Here's how the part is built. I have some questions about the finished solid (model axes, mm). A direction names the side the tool comes from. Round coordinates to 2 decimals unless told otherwise and drop trailing zeros. Write each loop counter-clockwise with the first axis right and the second up, starting at its lowest first coordinate (ties: lowest second). Pieces come first, ordered by that corner, then holes. Notation, with made-up numbers: (6, 79) -> (12, 79) arc R22 cw to (12, 117) -> close; hole circle Ø9 at (41.5, -30.75). An arc over 180 degrees is marked (long way). Answer in a Markdown table with one row per item.
from build123d import *

# Parameters (mm, degrees)
BOSS_EXTRUDE1_DEPTH = 12.5
SKETCH2_R           = 2
SKETCH2_R_2         = 0.5
BOSS_EXTRUDE2_DEPTH = 0.5
SKETCH2_2_R         = 0.5
BOSS_EXTRUDE3_DEPTH = 3
SKETCH2_4_R         = 2
BOSS_EXTRUDE4_DEPTH = 13.5
CUT_EXTRUDE1_START  = 12.5
SKETCH4_W           = 1.5
SKETCH4_H           = 2
CUT_EXTRUDE1_DEPTH  = 2
BOSS_EXTRUDE5_START = 12.5
SKETCH5_W           = 0.2
SKETCH5_H           = 1.5
BOSS_EXTRUDE5_DEPTH = 1.5
FILLET1_R           = 0.5
CUT_EXTRUDE2_START  = 12.5
CUT_EXTRUDE2_DEPTH  = 1


with BuildPart() as part:
    # Sketch1 → Boss-Extrude1 (new body)
    with BuildSketch(Plane.XY):
        with BuildLine():
            Line((-3, -4), (3, -4))
            ThreePointArc((3, -4), (5, 0), (3, 4))
            Line((3, 4), (-3, 4))
            ThreePointArc((-3, 4), (-5, 0), (-3, -4))
        make_face()
    extrude(amount=BOSS_EXTRUDE1_DEPTH)

    # Sketch2 → Boss-Extrude2 (add)
    with BuildSketch(Plane.XY):
        Circle(SKETCH2_R)
        Circle(SKETCH2_R_2, mode=Mode.SUBTRACT)
    extrude(amount=-BOSS_EXTRUDE2_DEPTH)

    # Sketch2<2> → Boss-Extrude3 (add)
    with BuildSketch(Plane.XY):
        Circle(SKETCH2_2_R)
    extrude(amount=-BOSS_EXTRUDE3_DEPTH)

    # Sketch2<4> → Boss-Extrude4 (add)
    with BuildSketch(Plane.XY):
        Circle(SKETCH2_4_R)
    extrude(amount=BOSS_EXTRUDE4_DEPTH)

    # Sketch4 → Cut-Extrude1 (cut)
    with BuildSketch(Plane.XY.offset(CUT_EXTRUDE1_START)):
        with Locations((0, 4)):
            Rectangle(SKETCH4_W, SKETCH4_H)
        with Locations((0, -4)):
            Rectangle(SKETCH4_W, SKETCH4_H)
    extrude(amount=-CUT_EXTRUDE1_DEPTH, mode=Mode.SUBTRACT)

    # Sketch5 → Boss-Extrude5 (add)
    with BuildSketch(Plane.XY.offset(BOSS_EXTRUDE5_START)):
        with Locations((3.1, 0)):
            Rectangle(SKETCH5_W, SKETCH5_H)
        with Locations((-3.1, 0)):
            Rectangle(SKETCH5_W, SKETCH5_H)
    extrude(amount=BOSS_EXTRUDE5_DEPTH)

    # Fillet1
    fillet1_edges = [part.edges().sort_by_distance(p)[0] for p in [
        (3.1, -0.75, 14),
        (3.1, 0.75, 14),
        (-3.1, -0.75, 14),
        (-3.1, 0.75, 14),
    ]]
    fillet(fillet1_edges, radius=FILLET1_R)

    # Sketch6 → Cut-Extrude2 (cut)
    with BuildSketch(Plane.XY.offset(CUT_EXTRUDE2_START)):
        with BuildLine():
            Line((-3, -4), (3, -4))
            ThreePointArc((3, -4), (5, 0), (3, 4))
            Line((3, 4), (-3, 4))
            ThreePointArc((-3, 4), (-5, 0), (-3, -4))
        make_face()
        with BuildLine():
            Line((-2.993325909, -3.98), (2.993325909, -3.98))
            ThreePointArc((2.993325909, -3.98), (4.98, 0), (2.993325909, 3.98))
            Line((2.993325909, 3.98), (-2.993325909, 3.98))
            ThreePointArc((-2.993325909, 3.98), (-4.98, 0), (-2.993325909, -3.98))
        make_face(mode=Mode.SUBTRACT)
    extrude(amount=-CUT_EXTRUDE2_DEPTH, mode=Mode.SUBTRACT)


solid = part.part
1) I need wall thicknesses on line 1 (Z direction, x = -1, y = 2.25); line 2 (Y direction, x = 0, z = -1.5); line 3 (Y direction, x = 4, z = 10). Which ranges of each line are inside material? Lowest first, please. Write a range as [from, to].
Response:
| item | result |
|---|---|
| line 1 | z = [0, 12.5] |
| line 2 | y = [-0.5, 0.5] |
| line 3 | y = [-3, 3] |
2) For pin 1 (1.5 mm diameter, centred on y = -3, z = 3, fed in from -X); pin 2 (0.8 mm diameter, centred on y = 0, z = 13, fed in from +X); pin 3 (0.5 mm diameter, centred on x = 1.5, z = 12, fed in from -Y); pin 4 (5 mm diameter, centred on x = -3.5, z = 11.5, fed in from +Y), each with a flat end and sliding along its axis, tell me the tip position at first contact or that it passes through.
Response:
| item | result |
|---|---|
| pin 1 | stops at x = -4.47 |
| pin 2 | stops at x = 3.2 |
| pin 3 | stops at y = -3.98 |
| pin 4 | stops at y = 4 |
3) We'd pull the mould along X, two halves only. Please class faces 1 (the face through (-3.2, 0, 13)), 2 (the face through (4.98, -0.06, 12.01)), 3 (the face through (0, -3.5, 10.5)), 4 (the face through (-0.108, -0.488, -1.732)): +X half, -X half, draft (parallel to the pull), parting line (faces both ways), or undercut.
Response:
| item | result |
|---|---|
| face 1 | -X half |
| face 2 | +X half |
| face 3 | undercut |
| face 4 | parting line |
4) I want a section at C-C, the plane z = 5. List the corners of the cut face in (x, y) for me, and give its area (3 significant figures).
Response:
| item | result |
|---|---|
| outline | (-3, -4) -> (3, -4) arc R5 ccw to (3, 4) -> (-3, 4) arc R5 ccw to start |
| area | 70.4 mm^2 |
5) I want a section at A-A, the plane x = 0. List the corners of the cut face in (y, z) for me, and give its area (4 significant figures).
Response:
| item | result |
|---|---|
| outline | (-4, 0) -> (-2, 0) -> (-2, -0.5) -> (-0.5, -0.5) -> (-0.5, -3) -> (0.5, -3) -> (0.5, -0.5) -> (2, -0.5) -> (2, 0) -> (4, 0) -> (4, 10.5) -> (3, 10.5) -> (3, 12.5) -> (2, 12.5) -> (2, 13.5) -> (-2, 13.5) -> (-2, 12.5) -> (-3, 12.5) -> (-3, 10.5) -> (-4, 10.5) -> close |
| area | 104.5 mm^2 |
6) Which directions (+Z, -Z, +X, -X, +Y, -Y) give clear straight access to the entire face, cutting with the end or side of a thin tool? Please do faces 5 (the face through (-0.75, -3.5, 11.5)), 6 (the face through (3, 0, 13)), 7 (the face through (0, 3.5, 10.5)).
Response:
| item | result |
|---|---|
| face 5 | +Z, -Y |
| face 6 | +Z, +Y, -Y |
| face 7 | +Z, +Y |
